For this review, take the finished solid that the model builds, in its own axes (mm). Give positions to 0.01 mm unless a question says otherwise; leave off trailing zeros. One line per item, written item: value.
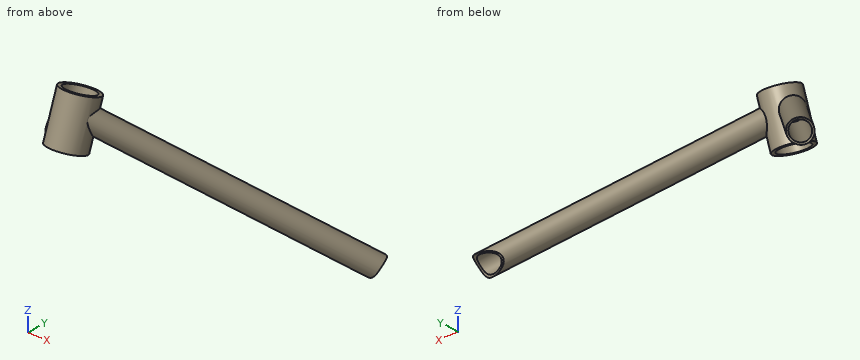
```python
from build123d import *

# Parameters (mm, degrees)
SKETCH1_R               = 15.875
BOSS_EXTRUDE1_DEPTH     = 20.701
SWEEP1_PROFILE_R        = 9.525
SWEEP2_PROFILE_R        = 9.525
CUT_EXTRUDE2_REACH      = 371.805
SKETCH36_R              = 7.9375
CUT_EXTRUDE3_REACH      = 371.805
CUT_EXTRUDE3_END_RADIUS = 15.875
SKETCH37_R              = 7.9375
SKETCH77_R              = 15.875
BOSS_EXTRUDE2_DEPTH     = 41.402
CUT_EXTRUDE1_REACH      = 251.445
SKETCH2_R               = 12.7
SKETCH83_R              = 12.7


with BuildPart() as part:
    # Sketch1 → Boss-Extrude1 (new, symmetric)
    with BuildSketch(Plane(origin=(0, 0, 0), x_dir=(1, 0, 0), z_dir=(0, 0.34202014332566943, 0.9396926207859081))):
        with Locations(Location((0, 0, 0), (0, 0, 270))):
            Circle(SKETCH1_R)
    extrude(amount=BOSS_EXTRUDE1_DEPTH, both=True)

    # Sweep1: sweep along a path in Sketch4
    with BuildLine(Plane(origin=(0, 3.144101118, 3.616874596), x_dir=(1, 0, 0), z_dir=(0, 0.6560590289905084, 0.754709580222771))) as sweep1_path:
        Line((-5.08, -4.165974834), (-143.483994092, 193.495413453))
    # Sweep1 profile (on start of the path) → Sweep1 (sweep)
    with BuildSketch(Plane(origin=(-5.08, 0, 6.35), x_dir=(0.7330812283825076, 0.6801410975622587, 0), z_dir=(-0.5735764363510472, 0.6182218954839692, -0.5374120947718255))):
        Circle(SWEEP1_PROFILE_R)
    sweep(path=sweep1_path.line)

    # Sweep2: sweep along a path in Sketch15
    with BuildLine(Plane(origin=(0, 3.144101118, 3.616874596), x_dir=(1, 0, 0), z_dir=(0, 0.6560590289905084, 0.754709580222771))) as sweep2_path:
        Line((5.08, -4.165974834), (143.483994092, 193.495413453))
    # Sweep2 profile (on start of the path) → Sweep2 (sweep)
    with BuildSketch(Plane(origin=(5.08, 0, 6.35), x_dir=(0.7330812283825074, -0.6801410975622589, 0), z_dir=(0.5735764363510474, 0.6182218954839692, -0.5374120947718254))):
        Circle(SWEEP2_PROFILE_R)
    sweep(path=sweep2_path.line)

    # Sketch36 → Cut-Extrude2 (cut, up to next)
    with BuildSketch(Plane(origin=(-138.117895022, 148.868575223, -129.409478119), x_dir=(0.8191108775847741, 0.4394391101382058, -0.36871484741361205), z_dir=(-0.5735764363510472, 0.6182218954839691, -0.5374120947718255)), mode=Mode.PRIVATE) as cut_extrude2_sk1:
        with Locations(Location((-6.502422539, -4.857839146, 0), (0, 0, 154.073467295))):
            Circle(SKETCH36_R)
    cut_extrude2_tool1 = extrude(cut_extrude2_sk1.sketch, amount=-CUT_EXTRUDE2_REACH, mode=Mode.PRIVATE) & part.part
    add(cut_extrude2_tool1.solids().sort_by_distance((-143.483994, 149.176943, -123.327538))[0], mode=Mode.SUBTRACT)

    # Cut-Extrude3: up to this cylinder (the profile starts outside it)
    cut_extrude3_end = Plane(origin=(0, -22.186319293, -60.956411279), z_dir=(0, -0.34202014332566943, -0.9396926207859081)) * Cylinder(CUT_EXTRUDE3_END_RADIUS, 776.36, mode=Mode.PRIVATE)
    # Sketch37 → Cut-Extrude3 (cut, up to the surface)
    with BuildSketch(Plane(origin=(138.117895022, 148.868575223, -129.409478119), x_dir=(0.8191108775847737, -0.4394391101382061, 0.36871484741361227), z_dir=(0.5735764363510476, 0.6182218954839689, -0.5374120947718255)), mode=Mode.PRIVATE) as cut_extrude3_sk1:
        with Locations(Location((6.502422539, -4.857839146, 0), (0, 0, 205.926532705))):
            Circle(SKETCH37_R)
    cut_extrude3_tool1 = extrude(cut_extrude3_sk1.sketch, amount=-CUT_EXTRUDE3_REACH, mode=Mode.PRIVATE) - cut_extrude3_end
    add(cut_extrude3_tool1.solids().sort_by_distance((143.483994, 149.176943, -123.327538))[0], mode=Mode.SUBTRACT)

    # Sketch77 → Boss-Extrude2 (add)
    with BuildSketch(Plane(origin=(0, 7.080158987, 19.452576943), x_dir=(1, 0, 0), z_dir=(0, 0.34202014332566943, 0.9396926207859082))):
        with Locations(Location((0, 0, 0), (0, 0, 270))):
            Circle(SKETCH77_R)
    extrude(amount=-BOSS_EXTRUDE2_DEPTH)

    # Sketch2 → Cut-Extrude1 (cut, up to next)
    with BuildSketch(Plane(origin=(0, -7.080158987, -19.452576943), x_dir=(-1, 0, 0), z_dir=(0, -0.34202014332566943, -0.9396926207859081)), mode=Mode.PRIVATE) as cut_extrude1_sk1:
        with Locations(Location((0, 0, 0), (0, 0, 90))):
            Circle(SKETCH2_R)
    cut_extrude1_tool1 = extrude(cut_extrude1_sk1.sketch, amount=-CUT_EXTRUDE1_REACH, mode=Mode.PRIVATE) & part.part
    add(cut_extrude1_tool1.solids().sort_by_distance((0, -7.080159, -19.452577))[0], mode=Mode.SUBTRACT)

    # Cut-Sweep1: sweep along a path in Sketch40
    with BuildLine(Plane(origin=(-106.934, 0, -127), x_dir=(1, 0, 0), z_dir=(0, 0, 1))) as cut_sweep1_path:
        Line((-63.663829669, 149.860844852), (100.20235662, 162.304768472))
        ThreePointArc((100.20235662, 162.304768472), (106.934, 162.56), (113.66564338, 162.304768472))
        Line((113.66564338, 162.304768472), (277.531829669, 149.860844852))
    # Sketch83 → Cut-Sweep1 (sweep, cut)
    with BuildSketch(Plane(origin=(170.597829669, 149.860844852, -127), x_dir=(0, 0, 1), z_dir=(-0.99712900418122, 0.07572152283577528, 0))):
        with Locations((0, -0.255231528)):
            Circle(SKETCH83_R)
    sweep(path=cut_sweep1_path.line, mode=Mode.SUBTRACT)


solid = part.part
```
(1) Take a section at A-A (y = 45). Give the number of separate pieces and of enclosed holes in the cut face, then the cut area to 3 significant figures.
Answers below:
separate pieces: 2
enclosed holes: 2
area: 282 mm^2
(2) Wall thickness on line 1 (X direction, y = 109, z = -95); line 2 (X direction, y = 118.5, z = -101); line 3 (Y direction, x = -91, z = -78): over which ranges is each line inside the solid? List them lowest first. Write a range as from..to.
Answers below:
line 1: x = -119.15..-116.79, -101.69..-99.33, 99.33..101.69, 116.79..119.15
line 2: x = -127.93..-125.84, -108.19..-106.1, 106.1..108.19, 125.84..127.93
line 3: y = 83.1..85.23, 104.12..106.26
(3) For P1, Ø1.5, axis at x = 91, y = 110.5, coming from the +Z side; P2, Ø12, axis at y = 24, z = -6.5, coming from the +X side; P3, Ø8, axis at y = 27, z = -27.5, coming from the -X side; P4, Ø1.5, axis at x = -93.5, z = -71.5, coming from the -Y side, all flat-tipped, find the tip position at first contact; note any pin that passes through.
Answers below:
P1: passes through
P2: stops at x = 38.32
P3: stops at x = -46.77
P4: stops at y = 80.72
